Verification items for the finished model (mm, model axes). A direction names the side the tool comes from. Give positions to 0.01 mm unless a question says otherwise; leave off trailing zeros. Loops run counter-clockwise (first coordinate to the right, second up) from the corner with the lowest first, then second, coordinate; pieces in that order, holes last. Notation, with made-up numbers: (71, 9.5) - (127, 9.5) arc R21 ccw to (127, 41.5) - close; hole circle Ø2 at (-26, 38). An arc over 180 degrees is marked (long way). Put each result on its own line as item: value. Start each with the question number.
Autodesk Inventor part; units mm, degrees
ref_plane "YZ Plane" through (0, 0, 0) normal (1, 0, 0) x (0, 1, 0)
ref_plane "XZ Plane" through (0, 0, 0) normal (0, 1, 0) x (-1, 0, 0)
ref_plane "XY Plane" through (0, 0, 0) normal (0, 0, 1) x (1, 0, 0)
sketch "Sketch1" plane through (0, 0, 0) normal (0, 1, 0) x (-1, 0, 0)
  line L0 (0, -6.35) -> (0, -98.0626)
  line L1 (10.8401, -102.5527) -> (102.5527, -10.8401)
  line L2 (98.0626, 0) -> (6.35, 0)
  arc A0 (102.5527, -10.8401) -> (98.0626, 0) centre (98.0626, -6.35) ccw
  arc A1 (0, -98.0626) -> (10.8401, -102.5527) centre (6.35, -98.0626) ccw
  arc A2 (6.35, 0) -> (0, -6.35) centre (6.35, -6.35) ccw
  line L3 (0, 0) -> (-20, 0)
  line L4 (-20, 0) -> (-20, -104.4126)
  line L5 (-20, -104.4126) -> (0, -104.4126)
  line L6 (0, -104.4126) -> (0, 0)
  line L7 (0, 0) -> (6.35, 0)
  line L8 (0, -104.4126) -> (6.35, -104.4126)
  point P0 (113.3929, 0)
  dimension "d0" = 113.3929
  dimension "d1" = 6.35
  dimension "d8" = 20
extrude "Extrusion1" add sketch "Sketch1" along normal blind 6.6929
sketch "Sketch2" plane through (0, 6.6929, 0) normal (0, 1, 0) x (1, 0, 0)
  arc A0 (-6.35, 104.4126) -> (-10.8401, 102.5527) centre (-6.35, 98.0626) ccw
  line L0 (-10.8401, 102.5527) -> (-102.5527, 10.8401)
  arc A1 (-102.5527, 10.8401) -> (-98.0626, 0) centre (-98.0626, 6.35) ccw
  line L1 (-4.7625, 4.7625) -> (-104.211, 4.7625)
  line L2 (-101.8952, 4.7625) -> (-4.7625, 101.8952)
  line L3 (-4.7625, 104.211) -> (-4.7625, 4.7625)
  line L4 (-98.0626, 0) -> (20, 0)
  line L5 (20, 0) -> (20, 104.4126)
  line L6 (20, 104.4126) -> (-6.35, 104.4126)
  line L7 (0, 0) -> (0, 104.4126)
  point P0 (0, 0)
extrude "Extrusion2" add sketch "Sketch2" along normal blind 20 contours L6 L7 L4 A1 L0 A0
sketch "Sketch3" plane through (0, 6.6929, 0) normal (0, 1, 0) x (1, 0, 0)
  circle A0 centre (10, 25.4) radius 2.4193
  circle A1 centre (10, 79.0126) radius 2.4193
  line L0 (20, 0) -> (20, 104.4126)
  line L1 (0, 0) -> (20, 0)
  dimension "d9" = 10
  dimension "d10" = 25.4
  dimension "d11" = 25.4
  dimension "d12" = 4.8387
extrude "Extrusion3" cut sketch "Sketch3" against normal blind 12.954
sketch "Sketch5" plane through (-102.5527, 0, -10.8401) normal (-0.7071068, 0, -0.7071068) x (-0.7071068, 0, 0.7071068)
  circle A0 centre (-24.3815, 16.6929) radius 2.3813
  line L0 (-138.6815, 6.6929) -> (-138.6815, 26.6929)
  line L1 (-129.7012, 26.6929) -> (0, 26.6929)
  line L2 (-129.7012, 0) -> (0, 0)
  line L3 (-152.8236, 6.6929) -> (-138.6815, 6.6929)
  line L4 (-78.9927, 0) -> (-152.8236, 0)
  point P0 (-64.8506, 0)
  dimension "d15" = 114.3
  dimension "d17" = 16.6929
  dimension "d18" = 6.6929
  dimension "d19" = 4.7625
extrude "Extrusion4" cut sketch "Sketch5" against normal up to surface (4.7625 mm away)
fillet "Fillet1" radius 3.175 11 edges at (-4.7625, 16.6929, -4.7625) (-101.8952, 16.6929, -4.7625) (-4.7625, 16.6929, -101.8952) (0, 16.6929, -104.4126) (-8.78, 0, -103.9292) (-56.6964, 0, -56.6964) (-103.9292, 0, -3.92) (-39.0313, 0, 0) (6.825, 0, -104.4126) (20, 0, -52.2063) (0, 16.6929, 0)
properties part number "Part1_3DPrint"
1) Depth check by flat-ended pin: P1, Ø6, axis at y = 12.5, z = -13, coming from the -X side; P2, Ø6, axis at x = -20, y = 22.5, coming from the -Z side; P3, Ø5, axis at y = 15, z = -50, coming from the -X side. Enter the tip coordinate at first touch or a pass-through.
2) Section check A-A, the plane x = 10. Enter the section's corners in (y, z) (3 decimals), plus the area to 3 significant figures.
3) Draft check along X on faces 1 (the face through (-53.933, 16.553, -52.725)), 2 (the face through (-38.2, 0.95, -0.91)), 3 (the face through (-56.698, 0.955, -55.414)). Enter one of: pulls with the +X half, pulls with the -X half, needs draft (parallel to the pull), parting line crosses it, or undercut.
4) Set-up check for faces 4 (the face through (-0.95, 16.83, -0.91)), 5 (the face through (-5.717, 16.833, -5.668)), 6 (the face through (-0.91, 16.83, -103.46)): record each of +Z, -Z, +X, -X, +Y, -Y from which the full face is reachable in a straight line by a thin tool's end or side.
5) Scan lines: line 1 along Z through (x, y) = (10, 5); line 2 along Z through (x, y) = (10, 2.5); line 3 along Y through (x, z) = (-6.5, -59.5). Record each from-to range of solid material in increasing order. Write a range as from..to.
Results are:
1. P1: stops at x = -103.26
1. P2: stops at z = -96.39
1. P3: stops at x = -65.89
2. outline: (0, -101.238) arc R3.175 ccw to (3.175, -104.413) - (6.693, -104.413) - (6.693, -81.432) - (0, -81.432) - close; (0, -76.593) - (6.693, -76.593) - (6.693, -27.819) - (0, -27.819) - close; (0, -22.981) - (6.693, -22.981) - (6.693, 0) - (3.175, 0) arc R3.175 ccw to (0, -3.175) - close
2. area: 630 mm2
3. face 1: undercut
3. face 2: needs draft
3. face 3: pulls with the -X half
4. face 4: +Z, +X, +Y
4. face 5: +Y
4. face 6: -Z, +X, +Y
5. line 1: z = -104.41..-81.43, -76.59..-27.82, -22.98..0
5. line 2: z = -104.34..-81.43, -76.59..-27.82, -22.98..-0.07
5. line 3: y = 0..6.69
